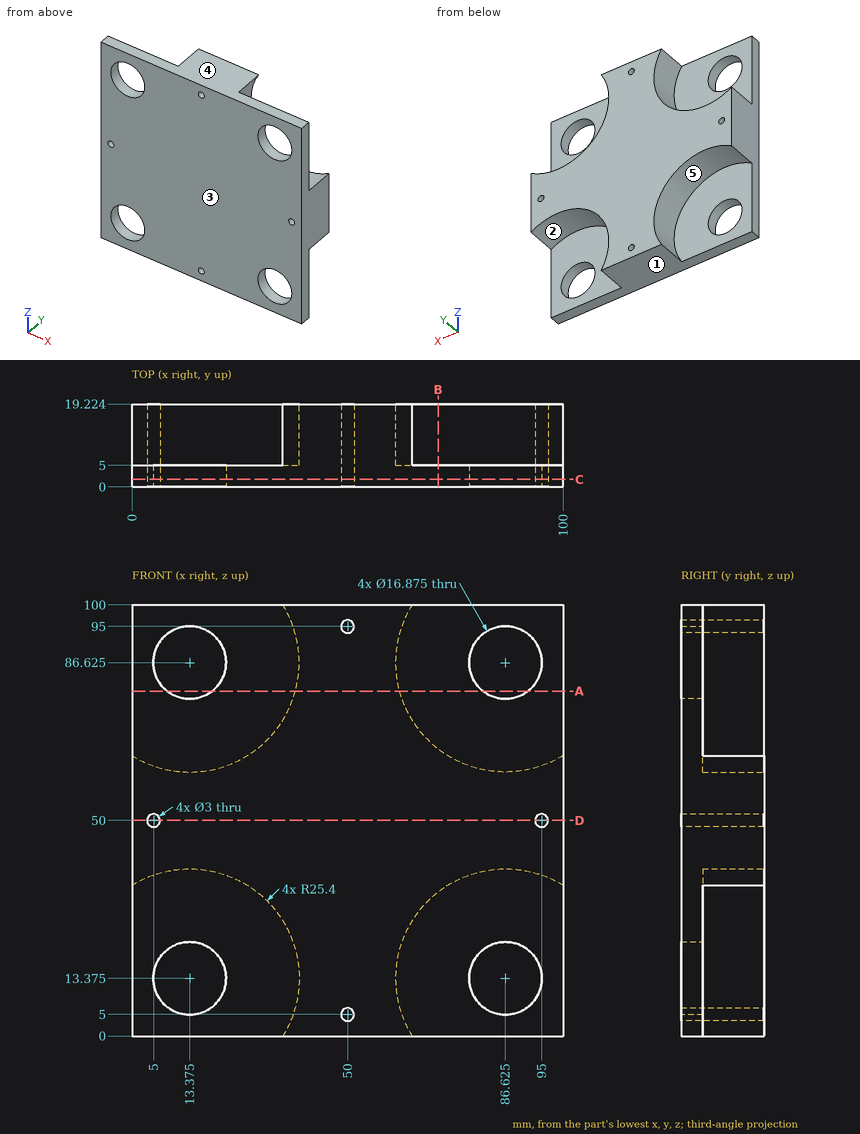
Answer from the drawing. Dimensions are ordinates in mm from the lowest x, y and z of the part. A direction names the side the tool comes from. Give positions to 0.01 mm unless a question says otherwise; leave off trailing zeros. Write each loop counter-clockwise with the first axis right and the second up, starting at its lowest first coordinate (ties: lowest second). Pieces come first, ordered by that corner, then holes.
1) Section B-B (x = 71) is taken. Write down the section's boundary in (y, z).
2) Section D-D (z = 50) is taken. Write down the section's boundary in (x, y), and give its area (3 significant figures).
3) Given P1, Ø2, axis at x = 77.5, z = 69, coming from the +Y side; P2, Ø4, axis at y = 16, z = 24, coming from the +X side; P3, Ø4, axis at y = 16.5, z = 18, coming from the +X side, each flat-ended and moving along its own axis, determine where each tip first touches the part or whether it passes through.
4) A tool of negligible diameter and unlimited length cuts with its end or side. For the marked faces 4 and 5, from which of +Z, -Z, +X, -X, +Y, -Y can it reach the whole face along a straight path? Write none if from no direction.
5) Section C-C (y = 1.75) is taken. Count the separate pieces of the cut face and the enclosed holes in it, and give its area (3 significant figures).
6) For a pull along Z with two mould halves and no side action, classify the marked faces 1, 2 and 3 as pulls with the +Z half, pulls with the -Z half, needs draft (parallel to the pull), parting line crosses it, or undercut.
7) Section A-A (z = 80) is taken. Write down the section's boundary in (x, y), and give its area (3 significant figures).
8) Find the intervals of material crossed by L1, parallel to X at y = 4.25, z = 16.5; L2, parallel to X at y = 5.75, z = 12.5; L3, parallel to Y at x = 29.5, z = 15, in increasing order.
Response:
1. outline: (0, 0) - (5, 0) - (5, 33.4) - (19.22, 33.4) - (19.22, 66.6) - (5, 66.6) - (5, 100) - (0, 100) - close
2. outline: (0, 0) - (3.5, 0) - (3.5, 19.22) - (0, 19.22) - close; (6.5, 0) - (93.5, 0) - (93.5, 19.22) - (6.5, 19.22) - close; (96.5, 0) - (100, 0) - (100, 19.22) - (96.5, 19.22) - close
2. area: 1,810 mm2
3. P1: stops at y = 5
3. P2: stops at x = 64.58
3. P3: stops at x = 62.1
4. face 4: +Z, +X, -X, +Y, -Y
4. face 5: +Y
5. separate pieces: 1
5. enclosed holes: 8
5. area: 9,080 mm2
6. face 1: pulls with the -Z half
6. face 2: undercut
6. face 3: needs draft
7. outline: (0, 0) - (8.15, 0) - (8.15, 5) - (0, 5) - close; (18.6, 0) - (81.4, 0) - (81.4, 5) - (62.1, 5) - (62.1, 19.22) - (37.9, 19.22) - (37.9, 5) - (18.6, 5) - close; (91.85, 0) - (100, 0) - (100, 5) - (91.85, 5) - close
7. area: 740 mm2
8. L1: x = 0 to 5.54, 21.21 to 78.79, 94.46 to 100
8. L2: x = 38.76 to 61.24
8. L3: y = 0 to 5
